from build123d import *

# Parameters (mm, degrees)
SKETCH268_R             = 4
PAD107_DEPTH            = 9.5
SKETCH269_R             = 7.5
PAD108_DEPTH            = 10
SKETCH270_R             = 1.5
POCKET131_DEPTH         = 7.501
BODY096_ROLL_ANGLE      = 90
BODY096_PLACEMENT_ANGLE = 180


with BuildPart() as part:
    # Sketch268 → Pad107 (new body)
    with BuildSketch(Plane.XY):
        Circle(SKETCH268_R)
        with BuildLine():
            Line((-1.245994, 1.5), (1.245994, 1.5))
            ThreePointArc((-1.245994, 1.5), (0, -1.95), (1.245994, 1.5))
        make_face(mode=Mode.SUBTRACT)
    extrude(amount=PAD107_DEPTH)

    # Sketch269 (on Face5 of Pad107) → Pad108 (join)
    with BuildSketch(Plane.XY.offset(9.5)):
        Circle(SKETCH269_R)
    extrude(amount=PAD108_DEPTH)

    # Sketch270 → Pocket131 (cut, through all)
    with BuildSketch(Plane.XZ):
        with Locations((0, 2.5)):
            Circle(SKETCH270_R)
    extrude(amount=-POCKET131_DEPTH, mode=Mode.SUBTRACT)


with BuildPart() as part_1:
    # Body096 roll: moved
    add(part.part.rotate(Axis((0, 0, 0), (1, 0, 0)), BODY096_ROLL_ANGLE))


with BuildPart() as part_2:
    # Body096 placement: moved
    add(part_1.part.moved(Location((-44.5, 20.5, 19))).rotate(Axis((-44.5, 20.5, 19), (0, 0, 1)), BODY096_PLACEMENT_ANGLE))


solid = part_2.part
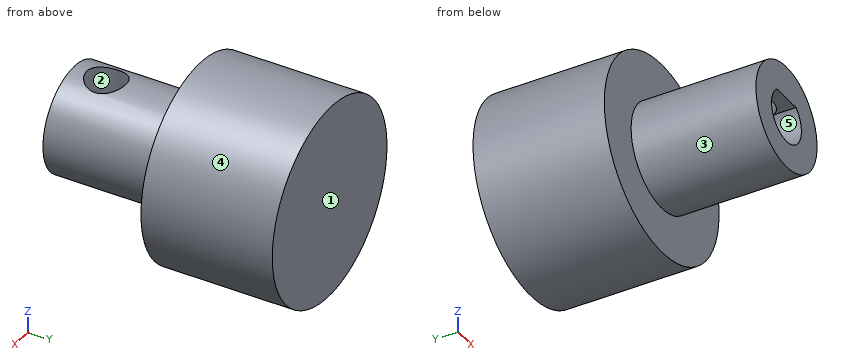
Verification items for the finished model (mm, model axes). Face numbers are marked on the shaded views. A direction names the side the tool comes from. Round coordinates to 2 decimals unless told otherwise and drop trailing zeros. Write each loop counter-clockwise with the first axis right and the second up, starting at its lowest first coordinate (ties: lowest second). Pieces come first, ordered by that corner, then holes.
(1) Section check D-D (y = 37.75). Enter the section's corners in (x, z), plus the area to 3 significant figures.
Returned:
outline: circle Ø15 at (-44.5, 19)
area: 177 mm2
(2) Section check A-A (x = -44.5). Enter the section's corners in (y, z), plus the area to 3 significant figures.
Returned:
outline: (20.5, 15) - (30, 15) - (30, 11.5) - (40, 11.5) - (40, 26.5) - (30, 26.5) - (30, 23) - (24.5, 23) - (24.5, 20.5) - (30, 20.5) - (30, 17.05) - (20.5, 17.05) - close; (20.5, 20.5) - (21.5, 20.5) - (21.5, 23) - (20.5, 23) - close
area: 186 mm2
(3) Access from +Z, -Z, +X, -X, +Y, -Y to the whole of each face (thin tool, end or side, straight path). Record for the marked faces 4 and 5.
Returned:
face 4: +Y, -Y
face 5: -Y
(4) Depth check by flat-ended pin: pin 1 Ø2.5 at (x, y) = (-45, 26.5) entering from -Z; pin 2 Ø8 at (x, y) = (-39.5, 32) entering from -Z; pin 3 Ø3 at (y, z) = (33, 24) entering from +X. Enter the tip coordinate at first touch or a pass-through.
Returned:
pin 1: stops at z = 15
pin 2: stops at z = 11.57
pin 3: stops at x = -37.87
(5) Section check B-B (z = 19). Enter the section's corners in (x, y).
Returned:
outline: (-52, 30) - (-48.5, 30) - (-48.5, 20.5) - (-46.45, 20.5) - (-46.45, 30) - (-42.55, 30) - (-42.55, 20.5) - (-40.5, 20.5) - (-40.5, 30) - (-37, 30) - (-37, 40) - (-52, 40) - close
(6) Mould release check, pull along X, two halves, no side actions. Record for the marked faces 1, 2 and 3: pulls with the +X half, pulls with the -X half, needs draft (parallel to the pull), parting line crosses it, or undercut.
Returned:
face 1: needs draft
face 2: undercut
face 3: parting line crosses it
(7) Section check C-C (y = 27.75). Enter the section's corners in (x, z), plus the area to 3 significant figures.
Returned:
outline: circle Ø8 at (-44.5, 19); hole (-45.75, 20.5) arc R1.95 ccw (long way) to (-43.25, 20.5) - close
area: 39.1 mm2
(8) Material ranges on line 1 (Y direction, x = -44.5, z = 21.1); line 2 (Z direction, x = -44.5, y = 26); line 3 (Y direction, x = -48.25, z = 15.5), recorded low to high.
Returned:
line 1: y = 20.5 to 21.5, 24.5 to 40
line 2: z = 15 to 17.05, 20.5 to 23
line 3: y = 30 to 40
